Geometry check sheet. Reference: drawing and pictorial views, mm from the part's lowest x, y, z. A direction names the side the tool comes from. Round coordinates to 2 decimals unless told otherwise and drop trailing zeros. Order: outer loops, then holes, each group sorted by start corner. A loop starts at its lowest first (then second) coordinate and runs counter-clockwise, first axis right, second up.
(1) Set-up check for the marked faces 1 and 2: record each of +Z, -Z, +X, -X, +Y, -Y from which the full face is reachable in a straight line by a thin tool's end or side.
(2) Go/stop test with flat-tipped pins: pin 1 (1 mm diameter, centred on x = 4.5, z = 1.5, fed in from -Y) (1 decimal); pin 2 (2 mm diameter, centred on x = 2.5, z = 3, fed in from +Y). Record where each tip stops, or that it passes through.
(3) Material ranges on line 1 along Y through (x, z) = (1.5, 7.25) (1 decimal); line 2 along Z through (x, y) = (3.25, 5.75) (1 decimal); line 3 along Y through (x, z) = (3, 4.75) (1 decimal), recorded low to high.
(4) Sectioned sample at B-B (z = 3.25). Record the boundary of the cut face in (x, y).
(5) Release check for a two-part mould opening along Y. For the marked faces 3, 4 and 5 record: +Y half, -Y half, draft (parallel to the pull), parting line (faces both ways), or undercut.
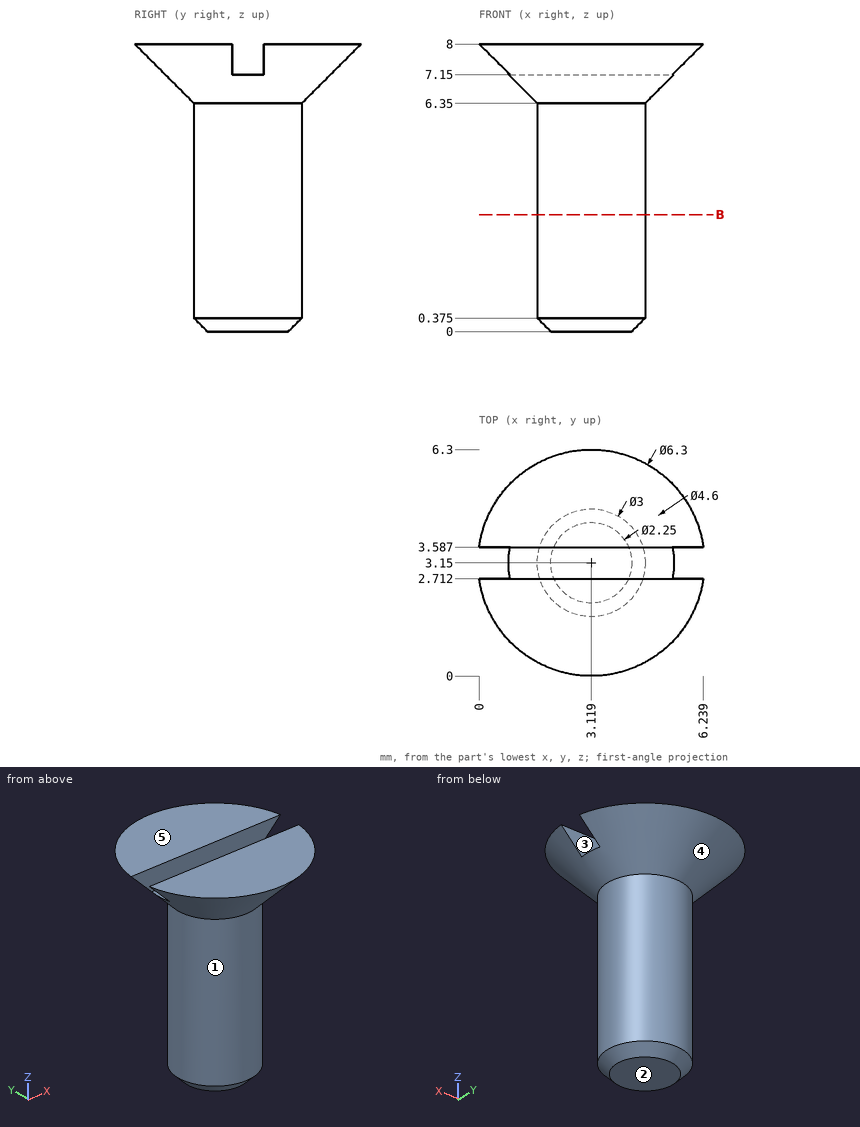
Answer below:
1. face 1: -Z
1. face 2: -Z, +X, -X, +Y, -Y
2. pin 1: stops at y = 1.9
2. pin 2: stops at y = 4.65
3. line 1: y = 1.4 to 2.7, 3.6 to 4.9
3. line 2: z = 7.5 to 8
3. line 3: y = 1.7 to 4.6
4. outline: circle Ø3 at (3.12, 3.15)
5. face 3: undercut
5. face 4: parting line
5. face 5: draft
